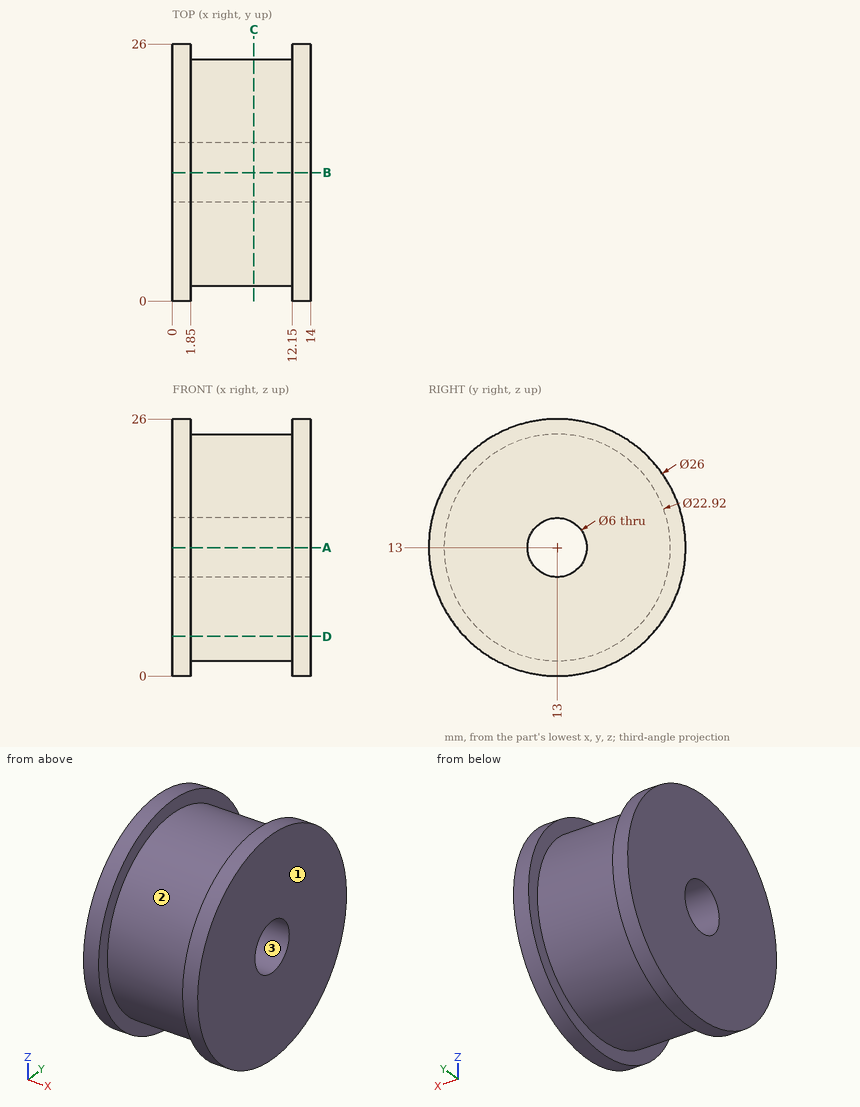
The figure shows three views and two pictorial views of one solid part (mm, origin at its lowest corner). Answer the questions. Round coordinates to 2 decimals unless told otherwise and drop trailing zeros. Write each loop counter-clockwise with the first axis right and the second up, starting at its lowest first coordinate (ties: lowest second). Pieces come first, ordered by that corner, then holes. Notation, with made-up numbers: (-3.5, -21.75) - (54.5, -21.75) arc R18 cw to (54.5, -7.75) - close; hole circle Ø3 at (48.5, 7). An arc over 180 degrees is marked (long way). One line per question, with ' | ' between items. Start each with the question number.
1. Find the intervals of material crossed by probe 1 along Y at (x, z) = (7.75, 13); probe 2 along X at (y, z) = (3.5, 4.25); probe 3 along Y at (x, z) = (11.25, 14.25), in increasing order. Write a range as [from, to].
2. For a pull along Y with two mould halves and no side action, classify the marked faces 1, 2 and 3 as +Y half, -Y half, draft (parallel to the pull), parting line (faces both ways), or undercut.
3. Section C-C (x = 8.25) is taken. Determine the outline of the cut face in (y, z).
4. Section D-D (z = 4) is taken. Determine the outline of the cut face in (x, y), and give its area (3 significant figures).
5. Section A-A (z = 13) is taken. Determine the outline of the cut face in (x, y), and give its area (3 significant figures).
6. Each of these flat-tipped pins is pushed along its axis until it touches: pin 1 (4 mm diameter, centred on x = 9, z = 3.5, fed in from +Y); pin 2 (3 mm diameter, centred on x = 4, y = 23, fed in from -Z); pin 3 (5 mm diameter, centred on y = 13, z = 13, fed in from +X); pin 4 (3 mm diameter, centred on x = 2.5, z = 6, fed in from -Y). Where does it stop, or does it pass through?
Filled in:
1) probe 1: [1.54, 10], [16, 24.46] | probe 2: [0, 1.85], [12.15, 14] | probe 3: [1.61, 10.27], [15.73, 24.39]
2) face 1: draft | face 2: parting line | face 3: undercut
3) outline: circle Ø22.92 at (13, 13); hole circle Ø6 at (13, 13)
4) outline: (0, 3.62) - (1.85, 3.62) - (1.85, 5.91) - (12.15, 5.91) - (12.15, 3.62) - (14, 3.62) - (14, 22.38) - (12.15, 22.38) - (12.15, 20.09) - (1.85, 20.09) - (1.85, 22.38) - (0, 22.38) - close | area: 216 mm²
5) outline: (0, 0) - (1.85, 0) - (1.85, 1.54) - (12.15, 1.54) - (12.15, 0) - (14, 0) - (14, 10) - (0, 10) - close; (0, 16) - (14, 16) - (14, 26) - (12.15, 26) - (12.15, 24.46) - (1.85, 24.46) - (1.85, 26) - (0, 26) - close | area: 248 mm²
6) pin 1: y = 21.66 | pin 2: z = 5.31 | pin 3: through | pin 4: y = 1.29
